```python
from build123d import *

# Parameters (mm, degrees)
F0_W           = 11
F0_H           = 9
F0_R           = 1.7
F1_DEPTH       = 5
F2_DEPTH       = 25
F4_D           = 5.5
F4_CBORE_D     = 9.75
F4_CBORE_DEPTH = 2
F5_DEPTH       = 5.001
F6_R           = 4
F7_ANGLE       = 90


# Not quite as in the source:
# - a feature names something its author has since deleted; it is built from what else it names


with BuildPart() as f1:
    # F0 (on Top) → F1 (new body)
    with BuildSketch(Plane.XY):
        with Locations((-48.0971363783, -35.5)):
            Rectangle(F0_W, F0_H)
        with Locations((-47.0971363783, -35.5)):
            Circle(F0_R, mode=Mode.SUBTRACT)
    extrude(amount=F1_DEPTH)



with BuildPart() as f1b:
    # F0 (on Top) → F1, piece 2 (new body)
    with BuildSketch(Plane.XY):
        with Locations((-48.0971363783, -4.5)):
            Rectangle(F0_W, F0_H)
        with Locations((-47.0971363783, -4.5)):
            Circle(F0_R, mode=Mode.SUBTRACT)
    extrude(amount=F1_DEPTH)


with BuildPart() as f1_1:
    add(f1.part)

    add(f1b.part)  # F2 merges F1b
    # F0 (on Top) → F2 (join)
    with BuildSketch(Plane.XY):
        Polygon((-58.5971363783, -40), (-53.5971363783, -40), (-53.5971363783, -31), (-53.5971363783, -9), (-53.5971363783, 0), (-58.5971363783, 0), align=None)
    extrude(amount=F2_DEPTH)

    # F4 (through all)
    with Locations(Plane.YZ.offset(-53.5971363783)):
        with Locations((-10, 15), (-30, 15)):
            CounterBoreHole(F4_D / 2, F4_CBORE_D / 2, F4_CBORE_DEPTH)

    # F3 (on face) → F5 (cut, through all)
    with BuildSketch(Plane.YZ.offset(-53.5971363783)):
        Polygon((-20, 15), (-31, 5), (-31, 0), (-9, 0), (-9, 5), align=None)
    extrude(amount=-F5_DEPTH, mode=Mode.SUBTRACT)

    # F6
    f6_edges = [f1_1.edges().sort_by_distance(p)[0] for p in [
        (-42.597136, 0, 2.5),
        (-42.597136, -40, 2.5),
        (-56.097136, -40, 25),
        (-56.097136, 0, 25),
        (-42.597136, -9, 2.5),
        (-42.597136, -31, 2.5),
        (-56.097136, -20, 15),
    ]]
    fillet(f6_edges, radius=F6_R)


with BuildPart() as f1_2:
    # F7: moved
    add(f1_1.part.rotate(Axis((-58.5971363783, -20, 0), (0, -1, 0)), F7_ANGLE))


solid = f1_2.part
```
Geometry check sheet. Reference: the model listing, model coordinates, mm. A direction names the side the tool comes from. Coordinates: 2 decimals unless noted, no trailing zeros. Order: outer loops, then holes, each group sorted by start corner. A loop starts at its lowest first (then second) coordinate and runs counter-clockwise, first axis right, second up. Notation, with made-up numbers: M 5.25,-28.75 L 38.25,-28.75 A10 ccw 38.25,-15.75 Z; hole C 28.25,57 d10. An arc over 180 degrees is marked long. Answer as a JSON object with one key per item and string values.
Q1. Cross-section at C-C on x = -66. Record the cut outline in (y, z), and give its area (3 significant figures).
Results are:
{"outline": "M -40,0 L -28.36,0 L -28.36,5 L -40,5 Z; M -11.64,0 L 0,0 L 0,5 L -11.64,5 Z", "area": "116 mm²"}
Q2. Cross-section at D-D on z = 7.25. Record the cut outline in (x, y).
Results are:
{"outline": "M -63.6,-40 L -58.6,-40 L -58.6,-31 L -63.6,-31 Z; M -63.6,-9 L -58.6,-9 L -58.6,0 L -63.6,0 Z"}
Q3. Cross-section at A-A on z = 11.5. Record the cut outline in (x, y), and give its area (3 significant figures).
Results are:
{"outline": "M -63.6,-40 L -58.6,-40 L -58.6,-37.2 L -63.6,-37.2 Z; M -63.6,-33.8 L -58.6,-33.8 L -58.6,-31 L -63.6,-31 Z; M -63.6,-9 L -58.6,-9 L -58.6,-6.2 L -63.6,-6.2 Z; M -63.6,-2.8 L -58.6,-2.8 L -58.6,0 L -63.6,0 Z", "area": "56.0 mm²"}
Q4. Tool access check on faces 1 (the flat face through (-63.597, -35, 9)), 2 (the flat face through (-61, -9, 6)), 3 (the cylindrical face through (-61.132, -7.859, 14.797)), 4 (the cylindrical face through (-82.394, -38.859, 2.535)). Record the directions out of +Z, -Z, +X, -X, +Y, -Y that give a thin tool (end or side, any length) a straight path to the whole face; none if there is none.
Results are:
{"face 1": "+Z, -X, +Y, -Y", "face 2": "+Z, -Z, +X", "face 3": "+Z, +X, -X", "face 4": "+Z, -Z, -X, -Y"}
Q5. Release check for a two-part mould opening along X. For faces 5 (the flat face through (-58.597, -4, 8)), 6 (the flat face through (-61.1, -4.5, 16)), 7 (the cylindrical face through (-78.43, -30.63, 4.01)) record: released by +X, released by -X, zero draft, split by the parting line, or undercut.
Results are:
{"face 5": "released by +X", "face 6": "zero draft", "face 7": "undercut"}
Q6. Scan lines: line 1 (Y direction, x = -60.6, z = 11.5); line 2 (Y direction, x = -75.25, z = 4); line 3 (Y direction, x = -65.5, z = 1.75). Record each from-to range of solid material in increasing order.
Results are:
{"line 1": "y = -40 to -37.2, -33.8 to -31, -9 to -6.2, -2.8 to 0", "line 2": "y = -40 to -34.59, -25.41 to -14.59, -5.41 to 0", "line 3": "y = -40 to -28.91, -11.09 to 0"}
Q7. Cross-section at B-B on y = -4.5. Record the cut outline in (x, z), and give its area (3 significant figures).
Results are:
{"outline": "M -83.6,0 L -58.6,0 L -58.6,9.8 L -63.6,9.8 L -63.6,5 L -83.6,5 Z; M -63.6,13.2 L -58.6,13.2 L -58.6,16 L -63.6,16 Z", "area": "163 mm²"}
Q8. Depth check by flat-ended pin: pin 1 Ø8 at (x, y) = (-73, -8) entering from +Z; pin 2 Ø9 at (x, y) = (-73.6, -30) entering from +Z; pin 3 Ø8 at (x, z) = (-76.5, 9.5) entering from -Y. Enter the tip coordinate at first touch or a pass-through.
Results are:
{"pin 1": "stops at z = 5", "pin 2": "stops at z = 3", "pin 3": "passes through"}
